Build history of the part. All positions in model axes, mm. A direction names the side the tool comes from. Round coordinates to 2 decimals unless told otherwise and drop trailing zeros. Write each loop counter-clockwise with the first axis right and the second up, starting at its lowest first coordinate (ties: lowest second). Pieces come first, ordered by that corner, then holes. Notation, with made-up numbers: (51.25, 64) -> (64.25, 64) arc R22 cw to (64.25, 92) -> close; hole circle Ø10 at (-17.5, -34.75). An arc over 180 degrees is marked (long way). Answer in a Markdown table with one row per item.
```python
from build123d import *

# Parameters (mm, degrees)
EXTRUDE_1_DEPTH     = 300
CUT_EXTRUDE_1_DEPTH = 290
CUT_EXTRUDE_3_DEPTH = 53
CUT_EXTRUDE_4_DEPTH = 60
CUT_EXTRUDE_5_DEPTH = 53
CUT_EXTRUDE_6_DEPTH = 60


with BuildPart() as part:
    # 草图1 → 拉伸1 (new body)
    with BuildSketch(Plane.XY):
        Polygon((0, 0), (0, 80), (5, 80), (25, 70), (25, 30), (5, 0), align=None)
    extrude(amount=EXTRUDE_1_DEPTH)

    # 草图2 → 切除-拉伸1 (cut)
    with BuildSketch(Plane(origin=(0, 80, 0), x_dir=(-1, 0, 0), z_dir=(0, 1, 0))):
        Polygon((0, 276.65), (-136.816544737, 333.321268387), (0, 333.321268387), align=None)
        Polygon((0, 0), (0, 23.35), (-107.528203225, -21.189640114), (0, -21.189640114), align=None)
    extrude(amount=-CUT_EXTRUDE_1_DEPTH, mode=Mode.SUBTRACT)

    # 草图5 → 切除-拉伸3 (cut)
    with BuildSketch(Plane.XY.offset(28.35)):
        Polygon((0, 75), (6.05572809, 75), (21, 67.527864045), (21, 31.211102551), (3.525931633, 5), (0, 5), align=None)
    extrude(amount=CUT_EXTRUDE_3_DEPTH, mode=Mode.SUBTRACT)

    # 草图6 → 切除-拉伸4 (cut)
    with BuildSketch(Plane.XY.offset(86.35)):
        Polygon((0, 75), (6.05572809, 75), (21, 67.527864045), (21, 31.211102551), (3.525931633, 5), (0, 5), align=None)
    extrude(amount=CUT_EXTRUDE_4_DEPTH, mode=Mode.SUBTRACT)

    # 草图7 → 切除-拉伸5 (cut)
    with BuildSketch(Plane.XY.offset(218.65)):
        Polygon((0, 75), (6.05572809, 75), (21, 67.527864045), (21, 31.211102551), (3.525931633, 5), (0, 5), align=None)
    extrude(amount=CUT_EXTRUDE_5_DEPTH, mode=Mode.SUBTRACT)

    # 草图8 → 切除-拉伸6 (cut)
    with BuildSketch(Plane.XY.offset(213.65)):
        Polygon((0, 75), (6.05572809, 75), (21, 67.527864045), (21, 31.211102551), (3.525931633, 5), (0, 5), align=None)
    extrude(amount=-CUT_EXTRUDE_6_DEPTH, mode=Mode.SUBTRACT)


solid = part.part
```
Q1. Saw through at C-C on z = 74. Write the cut outline in (x, y), plus the area to 3 significant figures.
A:
| item | result |
|---|---|
| outline | (0, 0) -> (5, 0) -> (25, 30) -> (25, 70) -> (5, 80) -> (0, 80) -> (0, 75) -> (6.06, 75) -> (21, 67.53) -> (21, 31.21) -> (3.53, 5) -> (0, 5) -> close |
| area | 415 mm² |
Q2. Two-plate mould, pull along Y, no slides. Class faces 1 (the flat face through (9.547, 40.56, 280.605)), 2 (the flat face through (21, 50, 184)), 3 (the flat face through (8, 40, 81.35)), 4 (the flat face through (15, 75, 148)): released by +Y, released by -Y, zero draft, split by the parting line, or undercut.
A:
| item | result |
|---|---|
| face 1 | zero draft |
| face 2 | undercut |
| face 3 | undercut |
| face 4 | released by +Y |
Q3. Wall check: line 1 (Z direction, x = 6.25, y = 60); line 2 (Z direction, x = 14.25, y = 24); line 3 (X direction, y = 33, z = 160.5). Give the ranges that are in metal, low to high. Write a range as [from, to].
A:
| item | result |
|---|---|
| line 1 | [20.76, 28.35], [81.35, 86.35], [146.35, 153.65], [213.65, 218.65], [271.65, 279.24] |
| line 2 | [17.45, 28.35], [81.35, 86.35], [146.35, 153.65], [213.65, 218.65], [271.65, 282.55] |
| line 3 | [21, 25] |
Q4. Saw through at A-A on x = 15.5. Write the cut outline in (y, z).
A:
| item | result |
|---|---|
| outline | (15.75, 16.93) -> (74.75, 16.93) -> (74.75, 283.07) -> (15.75, 283.07) -> close; hole (22.96, 28.35) -> (70.28, 28.35) -> (70.28, 81.35) -> (22.96, 81.35) -> close; hole (22.96, 86.35) -> (70.28, 86.35) -> (70.28, 146.35) -> (22.96, 146.35) -> close; hole (22.96, 153.65) -> (70.28, 153.65) -> (70.28, 213.65) -> (22.96, 213.65) -> close; hole (22.96, 218.65) -> (70.28, 218.65) -> (70.28, 271.65) -> (22.96, 271.65) -> close |
Q5. Which spindle directions (+Z, -Z, +X, -X, +Y, -Y) get a long thin tool onto all of the face, cutting with end or side? Do faces 5 (the flat face through (25, 50, 148)), 6 (the flat face through (13.42, 71.32, 244.78)). Say none if no direction does.
A:
| item | result |
|---|---|
| face 5 | +Z, -Z, +X, +Y, -Y |
| face 6 | -X |
Q6. Saw through at B-B on y = 50.5. Write the cut outline in (x, z), plus the area to 3 significant figures.
A:
| item | result |
|---|---|
| outline | (0, 23.35) -> (25, 12.99) -> (25, 287.01) -> (0, 276.65) -> (0, 271.65) -> (21, 271.65) -> (21, 218.65) -> (0, 218.65) -> (0, 213.65) -> (21, 213.65) -> (21, 153.65) -> (0, 153.65) -> (0, 146.35) -> (21, 146.35) -> (21, 86.35) -> (0, 86.35) -> (0, 81.35) -> (21, 81.35) -> (21, 28.35) -> (0, 28.35) -> close |
| area | 1,850 mm² |
Q7. Saw through at D-D on y = 26.5. Write the cut outline in (x, z).
A:
| item | result |
|---|---|
| outline | (0, 23.35) -> (22.67, 13.96) -> (22.67, 286.04) -> (0, 276.65) -> (0, 271.65) -> (17.86, 271.65) -> (17.86, 218.65) -> (0, 218.65) -> (0, 213.65) -> (17.86, 213.65) -> (17.86, 153.65) -> (0, 153.65) -> (0, 146.35) -> (17.86, 146.35) -> (17.86, 86.35) -> (0, 86.35) -> (0, 81.35) -> (17.86, 81.35) -> (17.86, 28.35) -> (0, 28.35) -> close |
Q8. Drop flat-ended pins along their axis: P1, Ø5, axis at y = 49.5, z = 176, coming from the -X side; P2, Ø8, axis at x = 22, z = 96.5, coming from the -Y side; P3, Ø3, axis at x = 19, y = 51.5, coming from the -Z side. Give the stop position or say it passes through.
A:
| item | result |
|---|---|
| P1 | x = 21 |
| P2 | y = 19.5 |
| P3 | z = 14.86 |
